from build123d import *

# Parameters (mm, degrees)
SKETCH1_W           = 52
SKETCH1_H           = 6
BOSS_EXTRUDE1_DEPTH = 3
SKETCH2_W           = 25
SKETCH2_H           = 4
BOSS_EXTRUDE2_DEPTH = 40
SKETCH3_R           = 1.6
CUT_EXTRUDE1_DEPTH  = 48.801673611
FILLET1_R           = 3
SKETCH5_R           = 1.4
CUT_EXTRUDE3_DEPTH  = 51.606323716
SKETCH6_W           = 17
SKETCH6_H           = 17
CUT_EXTRUDE4_DEPTH  = 51.606323716
CHAMFER1_SIZE       = 2
CUT_EXTRUDE5_DEPTH  = 51.408332645
FILLET2_R           = 1


with BuildPart() as part:
    # Sketch1 → Boss-Extrude1 (new body)
    with BuildSketch(Plane(origin=(0, 0, 0), x_dir=(1, 0, 0), z_dir=(0, 1, 0))):
        Rectangle(SKETCH1_W, SKETCH1_H)
    extrude(amount=BOSS_EXTRUDE1_DEPTH)

    # Sketch2 → Boss-Extrude2 (add)
    with BuildSketch(Plane(origin=(0, 3, 0), x_dir=(1, 0, 0), z_dir=(0, 1, 0))):
        with Locations((-7.5, -1)):
            Rectangle(SKETCH2_W, SKETCH2_H)
    extrude(amount=BOSS_EXTRUDE2_DEPTH)

    # Sketch3 → Cut-Extrude1 (cut, through all)
    with BuildSketch(Plane(origin=(0, 3, 0), x_dir=(1, 0, 0), z_dir=(0, 1, 0))):
        with Locations(Location((-23, 0, 0), (0, 0, 270))):
            Circle(SKETCH3_R)
        with Locations(Location((23, 0, 0), (0, 0, 270))):
            Circle(SKETCH3_R)
    extrude(amount=-CUT_EXTRUDE1_DEPTH, mode=Mode.SUBTRACT)

    # Fillet1
    fillet1_edges = [part.edges().sort_by_distance(p)[0] for p in [
        (26, 1.5, -3),
        (26, 1.5, 3),
        (-26, 1.5, 3),
        (-26, 1.5, -3),
    ]]
    fillet(fillet1_edges, radius=FILLET1_R - 0.0001)  # a hair under: the kernel refuses the full size

    # Sketch5 → Cut-Extrude3 (cut, through all)
    with BuildSketch(Plane.XY.offset(3)):
        with Locations((2, 40)):
            Circle(SKETCH5_R)
        with Locations((-17, 21)):
            Circle(SKETCH5_R)
    extrude(amount=-CUT_EXTRUDE3_DEPTH, mode=Mode.SUBTRACT)

    # Sketch6 → Cut-Extrude4 (cut, through all)
    with BuildSketch(Plane.XY.offset(3)):
        with Locations((-7.5, 30.5)):
            Rectangle(SKETCH6_W, SKETCH6_H)
    extrude(amount=-CUT_EXTRUDE4_DEPTH, mode=Mode.SUBTRACT)

    # Chamfer1
    chamfer1_edges = [part.edges().sort_by_distance(p)[0] for p in [
        (5, 3, 1),
        (-7.5, 3, -1),
    ]]
    chamfer(chamfer1_edges, length=CHAMFER1_SIZE - 0.0001)  # a hair under: the kernel refuses the full size

    # Sketch7 → Cut-Extrude5 (cut, through all)
    with BuildSketch(Plane(origin=(0, 0, -1), x_dir=(-1, 0, 0), z_dir=(0, 0, -1))):
        Polygon((-2, 19), (-2, 7.500243065), (15.342054098, 19), align=None)
        Polygon((17, 16.499756935), (-0.342054098, 5), (17, 5), align=None)
    extrude(amount=-CUT_EXTRUDE5_DEPTH, mode=Mode.SUBTRACT)

    # Fillet2
    fillet2_edges = [part.edges().sort_by_distance(p)[0] for p in [
        (-17, 5, 1),
        (-17, 16.499756935, 1),
        (0.342054098, 5, 1),
        (2, 7.500243065, 1),
        (2, 19, 1),
        (-15.342054098, 19, 1),
        (5, 43, 1),
        (-20, 43, 1),
    ]]
    fillet(fillet2_edges, radius=FILLET2_R)


solid = part.part
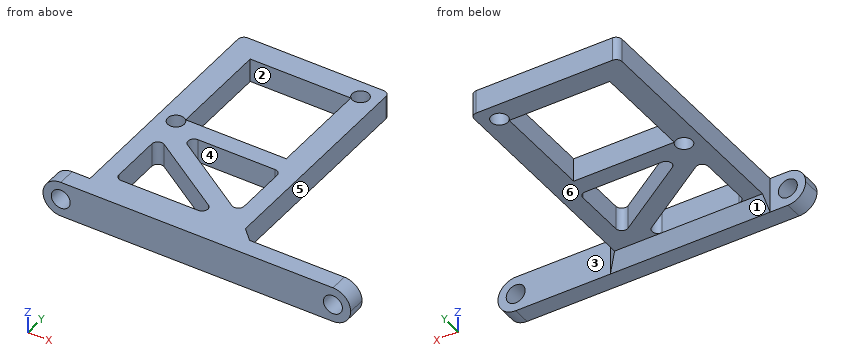
The model under review builds one solid part; all positions refer to its coordinate system, in mm. Face numbers are marked on the shaded views. A direction names the side the tool comes from. Give positions to 0.01 mm unless a question says otherwise; leave off trailing zeros. Order: outer loops, then holes, each group sorted by start corner. A loop starts at its lowest first (then second) coordinate and runs counter-clockwise, first axis right, second up. Notation, with made-up numbers: (20, 48.5) -> (39, 48.5) arc R21 ccw to (39, 73.5) -> close; hole circle Ø10 at (33, 64.25). An arc over 180 degrees is marked (long way). Write item = value, one per line. Start each with the question number.
(1) Tool access review of the marked faces 1, 2 and 3: name each direction out of +Z, -Z, +X, -X, +Y, -Y from which nothing blocks a thin tool from reaching the whole face with its end or side.
(2) Take a section at C-C (y = 11). Write out the cut boundary in (x, z).
(3) Take a section at D-D (y = 33). Write out the cut boundary in (x, z), plus the area to 3 significant figures.
(4) Draft analysis for pull direction X (two halves, no side actions). For the marked faces 4, 5 and 6, state which applies: +X half, -X half, draft (parallel to the pull), parting line (faces both ways), or undercut.
(5) Take a section at A-A (y = 40). Write out the cut boundary in (x, z), plus the area to 3 significant figures.
(6) Take a section at B-B (x = -11). State how many separate pieces and enclosed holes the cut face has, plus the area to 3 significant figures.
(7) For L1, parallel to X at y = 1.4, z = 0; L2, parallel to Y at x = -6, z = 1; L3, parallel to Y at x = -9, z = 2.5, list the stretches that pass through material, from the lowest coordinate up. Write a range as from..to.
(8) For pin 1 Ø2 at (y, z) = (34.5, 2) entering from -X; pin 2 Ø4.5 at (x, y) = (2, 40) entering from -Z; pin 3 Ø2.5 at (x, z) = (-23, 0) entering from +Y; pin 4 Ø2 at (y, z) = (14.5, 0.5) entering from +X, all flat-tipped, find the tip position at first contact; note any pin that passes through.
Returned:
q1.face_1 = -Z, +X, -X, +Y
q1.face_2 = +Z, -Z
q1.face_3 = +Z, -Z, +Y
q2.outline = (-20, -1) -> (-17, -1) -> (-17, 3) -> (-20, 3) -> close; (-8.71, -1) -> (-3.28, -1) -> (-3.28, 3) -> (-8.71, 3) -> close; (2, -1) -> (5, -1) -> (5, 3) -> (2, 3) -> close
q3.outline = (-20, -1) -> (-16, -1) -> (-16, 3) -> (-20, 3) -> close; (1, -1) -> (5, -1) -> (5, 3) -> (1, 3) -> close
q3.area = 32.0 mm²
q4.face_4 = undercut
q4.face_5 = +X half
q4.face_6 = draft
q5.outline = (-20, -1) -> (0.6, -1) -> (0.6, 3) -> (-20, 3) -> close; (3.4, -1) -> (5, -1) -> (5, 3) -> (3.4, 3) -> close
q5.area = 88.8 mm²
q6.separate_pieces = 4
q6.enclosed_holes = 0
q6.area = 70.4 mm²
q7.L1 = -26..-24.6, -21.4..21.4, 24.6..26
q7.L2 = 0..5, 9.21..12.81, 19..22, 39..43
q7.L3 = 0..5, 11.19..14.79, 19..22, 39..43
q8.pin_1 = -20
q8.pin_2 = -1
q8.pin_3 = through
q8.pin_4 = 5
